Check sheet for the modelled part. Datum: model origin and axes. Units: mm. Coordinates: 2 decimals unless noted, no trailing zeros. Order: outer loops, then holes, each group sorted by start corner. A loop starts at its lowest first (then second) coordinate and runs counter-clockwise, first axis right, second up. Notation, with made-up numbers: (74, 58) -> (86, 58) arc R29 ccw to (86, 88) -> close; hole circle Ø11 at (84, 18). An arc over 180 degrees is marked (long way). Put each result on its own line as item: value. Start each with the question number.
Autodesk Fusion 360 part; units mm, degrees
sketch "Sketch1" plane through (0, 0, 0) normal (0, 1, 0) x (1, 0, 0)
  line L0 (0, 22) -> (0, -20)
  line L1 (0, -20) -> (0, 22)
  line L2 (0, 22) -> (5, 22)
  line L3 (5, 22) -> (6, 2)
  line L4 (6, 2) -> (5.5, 12)
  spline S0 degree 5 poles (6, 2) (5.9827, 1.7824) (5.9481, 1.3582) (5.8959, 0.7544) (5.8257, 0.0148) (5.7362, -0.8023) (5.643, -1.5196) (5.5418, -2.1553) (5.4257, -2.7407) (5.2839, -3.328) (5.1043, -3.9784) (4.8788, -4.7424) (4.6082, -5.6399) (4.3058, -6.6446) (4.0057, -7.6551) (3.7526, -8.5268) (3.5809, -9.1453) (3.5015, -9.4723) (3.4752, -9.6361) (3.4126, -9.9335) (3.2758, -10.4901) (3.0887, -11.2035) (2.9025, -11.8965) (2.7579, -12.4288) (2.6805, -12.7125) knots 0 0 0 0 0 0 0.05 0.1 0.15 0.2 0.25 0.3 0.35 0.4 0.45 0.5 0.55 0.6 0.65 0.7 0.75 0.8 0.85 0.9 0.95 1 1 1 1 1 1
  spline S1 degree 5 poles (2.6805, -12.7125) (2.6817, -12.7823) (2.6847, -12.926) (2.6912, -13.1546) (2.7041, -13.487) (2.731, -13.9707) (2.7665, -14.447) (2.8048, -14.8795) (2.8364, -15.2067) (2.8538, -15.38) knots 0 0 0 0 0 0 0.2 0.4 0.6 0.8 1 1 1 1 1 1
  line L5 (2.8056, -14.8983) -> (2.9019, -15.8617)
  line L6 (3.6055, -8.9902) -> (3.3945, -10.0098)
  line L7 (2.8538, -15.38) -> (3, -15.38)
  line L8 (3, -15.38) -> (3, -16.4418)
  line L9 (3, -16.4418) -> (2.5935, -16.9599)
  spline S2 degree 5 poles (2.5935, -16.9599) (2.4709, -16.9161) (2.2311, -16.8356) (1.888, -16.7364) (1.459, -16.6412) (0.9544, -16.5633) (0.5663, -16.5212) (0.281, -16.4972) (0.0933, -16.4844) (0, -16.4788) knots 0 0 0 0 0 0 0.2 0.4 0.6 0.8 1 1 1 1 1 1
  line L10 (2.9043, -17.0709) -> (2.2828, -16.8488)
  point P0 (5.5, -2.3487)
  point P1 (4.5, -6)
  point P2 (3.5, -9.5)
revolve "Revolve1" add sketch "Sketch1" angle 360 about axis through (0, 0, -22) along (0, 0, 1)
fillet "Fillet1" radius 2 1 faces at (-0.3379, -0.3642, -22)
shell "Shell1" thickness 1 removed faces 1 at (0.3369, 1.7219, 16.7123)
1) Sectioned sample at B-B (z = -4.5). Record the boundary of the cut face in (x, y) (3 decimals).
2) Gauge pin test, flat ends, axial feed: pin 1 (4 mm diameter, centred on y = 1, z = 11, fed in from +X); pin 2 (4 mm diameter, centred on y = -4.5, z = -10.5, fed in from +X); pin 3 (1.1 mm diameter, centred on x = 0, y = 0, fed in from +Z). Record the tip position at first contact, or that the pin passes through.
3) Scan lines: line 1 along Y through (x, z) = (-2.5, -5); line 2 along Y through (x, z) = (-1.75, -15); line 3 along X through (y, z) = (0.5, 14). Record each from-to range of solid material in increasing order. Write a range as [from, to].
4) Sectioned sample at A-A (z = -15). Record the boundary of the cut face in (x, y), plus the area to 3 significant figures.
5) Mould release check, pull along X, two halves, no side actions. Record for faces 1 (the flat face through (0, 0, -22)), 2 (the cylindrical face through (-3, 0, 16)), 3 (the flat face through (0, 0, 16.38)): +X half, -X half, draft (parallel to the pull), parting line (faces both ways), or undercut.
Entries:
1. outline: circle Ø11.75 at (0, 0)
2. pin 1: stops at x = 3.58
2. pin 2: stops at x = 4.99
2. pin 3: stops at z = 16.38
3. line 1: y = [-5.29, 5.29]
3. line 2: y = [-5.06, 5.06]
3. line 3: x = [-2.69, 2.69]
4. outline: circle Ø10.7 at (0, 0)
4. area: 89.9 mm2
5. face 1: draft
5. face 2: parting line
5. face 3: undercut
